Part model, mm, in its own coordinate system. A direction names the side the tool comes from. Give positions to 0.01 mm unless a question says otherwise; leave off trailing zeros. Write each loop counter-clockwise with the first axis right and the second up, starting at its lowest first coordinate (ties: lowest second). Pieces come first, ordered by that corner, then holes. Notation, with made-up numbers: (66.25, 23) - (111.25, 23) arc R28 cw to (111.25, 62) - close; hole circle Ø9 at (-39, -20). An arc over 180 degrees is marked (long way). Answer as a JSON object with one key per item and string values. Group by question number.
```python
from build123d import *

# Parameters (mm, degrees)
SKETCH_1_W          = 37.4
SKETCH_1_H          = 27.4
EXTRUDE_1_DEPTH     = 5
FILLET_1_R          = 3
SHELL_1_T           = -1
SKETCH_2_W          = 25.4
SKETCH_2_H          = 17.4
CUT_EXTRUDE_1_DEPTH = 10
EXTRUDE_2_DEPTH     = 2
SKETCH_4_R          = 1
CUT_EXTRUDE_2_DEPTH = 24.714552494


with BuildPart() as part:
    # 草图1 → 凸台-拉伸1 (new body)
    with BuildSketch(Plane.XY):
        Rectangle(SKETCH_1_W, SKETCH_1_H)
    extrude(amount=EXTRUDE_1_DEPTH)

    # 圆角1
    fillet_1_edges = [part.edges().sort_by_distance(p)[0] for p in [
        (18.7, -13.7, 2.5),
        (-18.7, -13.7, 2.5),
        (-18.7, 13.7, 2.5),
        (18.7, 13.7, 2.5),
    ]]
    fillet(fillet_1_edges, radius=FILLET_1_R)

    # 抽壳1
    shell_1_openings = [part.faces().sort_by_distance(p)[0] for p in [
        (0, 0, 5),
    ]]
    offset(amount=SHELL_1_T, openings=shell_1_openings, kind=Kind.INTERSECTION)

    # 草图2 → 切除-拉伸1 (cut)
    with BuildSketch(Plane(origin=(0, 0, 0), x_dir=(-1, 0, 0), z_dir=(0, 0, -1))):
        with Locations((0, 1)):
            Rectangle(SKETCH_2_W, SKETCH_2_H)
    extrude(amount=-CUT_EXTRUDE_1_DEPTH, mode=Mode.SUBTRACT)

    # 草图3 → 凸台-拉伸2 (add)
    with BuildSketch(Plane.XY.offset(1)):
        with BuildLine():
            Line((-17.7, -7.7), (-14.2, -7.7))
            ThreePointArc((-14.2, -7.7), (-13.139339828, -8.139339828), (-12.7, -9.2))
            Line((-12.7, -9.2), (-12.7, -12.7))
            Line((-12.7, -12.7), (-17.7, -12.7))
            Line((-17.7, -12.7), (-17.7, -7.7))
        make_face()
        with BuildLine():
            Line((12.7, -9.2), (12.7, -12.7))
            Line((12.7, -12.7), (17.7, -12.7))
            Line((17.7, -12.7), (17.7, -7.7))
            Line((17.7, -7.7), (14.2, -7.7))
            ThreePointArc((14.2, -7.7), (13.139339828, -8.139339828), (12.7, -9.2))
        make_face()
        with BuildLine():
            Line((17.7, 7.7), (14.2, 7.7))
            ThreePointArc((14.2, 7.7), (13.139339828, 8.139339828), (12.7, 9.2))
            Line((12.7, 9.2), (12.7, 12.7))
            Line((12.7, 12.7), (17.7, 12.7))
            Line((17.7, 12.7), (17.7, 7.7))
        make_face()
        with BuildLine():
            Line((-12.7, 9.2), (-12.7, 12.7))
            Line((-12.7, 12.7), (-17.7, 12.7))
            Line((-17.7, 12.7), (-17.7, 7.7))
            Line((-17.7, 7.7), (-14.2, 7.7))
            ThreePointArc((-14.2, 7.7), (-13.139339828, 8.139339828), (-12.7, 9.2))
        make_face()
    extrude(amount=EXTRUDE_2_DEPTH)

    # 草图4 → 切除-拉伸2 (cut, through all)
    with BuildSketch(Plane(origin=(0, 0, 0), x_dir=(-1, 0, 0), z_dir=(0, 0, -1))):
        with Locations((14.5, -9.5)):
            Circle(SKETCH_4_R)
        with Locations((14.5, 9.5)):
            Circle(SKETCH_4_R)
        with Locations((-14.5, 9.5)):
            Circle(SKETCH_4_R)
        with Locations((-14.5, -9.5)):
            Circle(SKETCH_4_R)
    extrude(amount=-CUT_EXTRUDE_2_DEPTH, mode=Mode.SUBTRACT)


solid = part.part
```
1) Band-saw the part on C-C (z = 1.9). List the corners of the cut face in (x, y), plus the area to 3 significant figures.
2) Band-saw the part on D-D (z = 4.25). List the corners of the cut face in (x, y), plus the area to 3 significant figures.
3) Mould opens along X. For faces 4 (the cylindrical face through (13.546, 9.8, 1.479)), 5 (the flat face through (18.7, 0, 2)), 6 (the cylindrical face through (-17.84, 12.8, 2.54)) say: pulls with the +X half, pulls with the -X half, needs draft (parallel to the pull), parting line crosses it, or undercut.
4) Band-saw the part on A-A (x = -10). List the corners of the cut face in (y, z), plus the area to 3 significant figures.
5) Which spindle directions (+Z, -Z, +X, -X, +Y, -Y) get a long thin tool onto all of the face, cutting with end or side? Do faces 1 (the flat face through (0.2, 9.7, 0.5)), 2 (the cylindrical face through (-17.84, -12.8, 2.54)), 3 (the cylindrical face through (-13.15, 8.13, 1.99)). Say none if no direction does.
6) Drop flat-ended pins along their axis: P1, Ø1.5, axis at x = -15, y = 9.5, coming from the +Z side; P2, Ø1.2, axis at x = 14.5, y = 9.5, coming from the +Z side; P3, Ø10, axis at x = -5, y = -5, coming from the +Z side. Give the stop position or say it passes through.
7) Band-saw the part on B-B (y = -3.75). List the corners of the cut face in (x, z).
8) Probe line 1 (Y direction, x = -14.5, z = 0.7); line 2 (Y direction, x = -14.5, z = 2.3); line 3 (Y direction, x = 7, z = 2.5). List the from-to ranges inside material, lowest first.
Verdict:
{
 "1": {"outline": "(-18.7, -10.7) arc R3 ccw to (-15.7, -13.7) - (15.7, -13.7) arc R3 ccw to (18.7, -10.7) - (18.7, 10.7) arc R3 ccw to (15.7, 13.7) - (-15.7, 13.7) arc R3 ccw to (-18.7, 10.7) - close; hole (-17.7, -7.7) - (-14.2, -7.7) arc R1.5 cw to (-12.7, -9.2) - (-12.7, -12.7) - (12.7, -12.7) - (12.7, -9.2) arc R1.5 cw to (14.2, -7.7) - (17.7, -7.7) - (17.7, 7.7) - (14.2, 7.7) arc R1.5 cw to (12.7, 9.2) - (12.7, 12.7) - (-12.7, 12.7) - (-12.7, 9.2) arc R1.5 cw to (-14.2, 7.7) - (-17.7, 7.7) - close; hole circle Ø2 at (-14.5, -9.5); hole circle Ø2 at (-14.5, 9.5); hole circle Ø2 at (14.5, -9.5); hole circle Ø2 at (14.5, 9.5)", "area": "203 mm2"},
 "2": {"outline": "(-18.7, -10.7) arc R3 ccw to (-15.7, -13.7) - (15.7, -13.7) arc R3 ccw to (18.7, -10.7) - (18.7, 10.7) arc R3 ccw to (15.7, 13.7) - (-15.7, 13.7) arc R3 ccw to (-18.7, 10.7) - close; hole (-17.7, -10.7) arc R2 ccw to (-15.7, -12.7) - (15.7, -12.7) arc R2 ccw to (17.7, -10.7) - (17.7, 10.7) arc R2 ccw to (15.7, 12.7) - (-15.7, 12.7) arc R2 ccw to (-17.7, 10.7) - close", "area": "121 mm2"},
 "3": {"face 4": "undercut", "face 5": "pulls with the +X half", "face 6": "pulls with the -X half"},
 "4": {"outline": "(-13.7, 0) - (-7.7, 0) - (-7.7, 1) - (-12.7, 1) - (-12.7, 5) - (-13.7, 5) - close; (9.7, 0) - (13.7, 0) - (13.7, 5) - (12.7, 5) - (12.7, 1) - (9.7, 1) - close", "area": "18.0 mm2"},
 "5": {"face 1": "+Z, -Z", "face 2": "+Z, -Z, -X, -Y", "face 3": "+Z"},
 "6": {"P1": "z = 3", "P2": "through", "P3": "z = 1"},
 "7": {"outline": "(-18.7, 0) - (-12.7, 0) - (-12.7, 1) - (-17.7, 1) - (-17.7, 5) - (-18.7, 5) - close; (12.7, 0) - (18.7, 0) - (18.7, 5) - (17.7, 5) - (17.7, 1) - (12.7, 1) - close"},
 "8": {"line 1": "-13.7 to -10.5, -8.5 to 8.5, 10.5 to 13.7", "line 2": "-13.7 to -10.5, -8.5 to -7.7, 7.7 to 8.5, 10.5 to 13.7", "line 3": "-13.7 to -12.7, 12.7 to 13.7"}
}
